```python
from build123d import *

# Parameters (mm, degrees)
EXTRUDE_1_DEPTH   = 7
SKETCH_1_W        = 4.5
SKETCH_1_H        = 2
EXTRUDE_1_2_DEPTH = 7
EXTRUDE_1_3_DEPTH = 7
EXTRUDE_1_4_DEPTH = 7
EXTRUDE_1_5_DEPTH = 7
EXTRUDE_1_6_DEPTH = 7
EXTRUDE_1_7_DEPTH = 7
EXTRUDE_2_DEPTH   = 3
SKETCH_3_W        = 21.86
SKETCH_3_H        = 15
EXTRUDE_3_DEPTH   = 5
FILLET_1_R        = 2
CHAMFER_1_SIZE    = 0.5


with BuildPart() as part:
    # Sketch 1 → Extrude 1 (new body)
    with BuildSketch(Plane(origin=(0, 0, 0), x_dir=(1, 0, 0), z_dir=(0, 1, 0))):
        Polygon((-0.13, 3.475), (-0.13, 1.525), (-2.19, 1.525), (-2.19, -1.525), (-0.13, -1.525), (-0.13, -3.475), (-2.19, -3.475), (-2.19, -6.525), (-0.13, -6.525), (-0.13, -7.495), (1.67, -7.495), (1.67, 7.505), (-0.13, 7.505), (-0.13, 6.525), (-2.19, 6.525), (-2.19, 3.475), align=None)
    extrude(amount=EXTRUDE_1_DEPTH)

    # Sketch 2 → Extrude 2 (add)
    with BuildSketch(Plane(origin=(0, 7, 0), x_dir=(1, 0, 0), z_dir=(0, 1, 0))):
        Polygon((-0.13, 7.505), (-0.13, 6.525), (-2.19, 6.525), (-2.19, 3.475), (-0.13, 3.475), (-0.13, 1.525), (-2.19, 1.525), (-2.19, -1.525), (-0.13, -1.525), (-0.13, -3.475), (-2.19, -3.475), (-2.19, -6.525), (-0.13, -6.525), (-0.13, -7.495), (1.67, -7.495), (1.67, 7.505), align=None)
    extrude(amount=EXTRUDE_2_DEPTH)



with BuildPart() as body_2:
    # Sketch 1 → Extrude 1 2 (new body)
    with BuildSketch(Plane(origin=(0, 0, 0), x_dir=(1, 0, 0), z_dir=(0, 1, 0))):
        with Locations((-7.44, 4)):
            Rectangle(SKETCH_1_W, SKETCH_1_H)
    extrude(amount=EXTRUDE_1_2_DEPTH)


with BuildPart() as body_3:
    # Sketch 1 → Extrude 1 3 (new body)
    with BuildSketch(Plane(origin=(0, 0, 0), x_dir=(1, 0, 0), z_dir=(0, 1, 0))):
        with Locations((-7.44, 0)):
            Rectangle(SKETCH_1_W, SKETCH_1_H)
    extrude(amount=EXTRUDE_1_3_DEPTH)


with BuildPart() as body_4:
    # Sketch 1 → Extrude 1 4 (new body)
    with BuildSketch(Plane(origin=(0, 0, 0), x_dir=(1, 0, 0), z_dir=(0, 1, 0))):
        with Locations((-7.44, -4)):
            Rectangle(SKETCH_1_W, SKETCH_1_H)
    extrude(amount=EXTRUDE_1_4_DEPTH)


with BuildPart() as body_5:
    # Sketch 1 → Extrude 1 5 (new body)
    with BuildSketch(Plane(origin=(0, 0, 0), x_dir=(1, 0, 0), z_dir=(0, 1, 0))):
        with Locations((6.92, 4)):
            Rectangle(SKETCH_1_W, SKETCH_1_H)
    extrude(amount=EXTRUDE_1_5_DEPTH)


with BuildPart() as body_6:
    # Sketch 1 → Extrude 1 6 (new body)
    with BuildSketch(Plane(origin=(0, 0, 0), x_dir=(1, 0, 0), z_dir=(0, 1, 0))):
        with Locations((6.92, 0)):
            Rectangle(SKETCH_1_W, SKETCH_1_H)
    extrude(amount=EXTRUDE_1_6_DEPTH)


with BuildPart() as body_7:
    # Sketch 1 → Extrude 1 7 (new body)
    with BuildSketch(Plane(origin=(0, 0, 0), x_dir=(1, 0, 0), z_dir=(0, 1, 0))):
        with Locations((6.92, -4)):
            Rectangle(SKETCH_1_W, SKETCH_1_H)
    extrude(amount=EXTRUDE_1_7_DEPTH)


with BuildPart() as part_1:
    add(part.part)

    add(body_2.part)  # Extrude 3 merges body 2

    add(body_3.part)  # Extrude 3 merges body 3

    add(body_4.part)  # Extrude 3 merges body 4

    add(body_5.part)  # Extrude 3 merges body 5

    add(body_6.part)  # Extrude 3 merges body 6

    add(body_7.part)  # Extrude 3 merges body 7
    # Sketch 3 → Extrude 3 (add)
    with BuildSketch(Plane.XZ):
        with Locations((-0.26, -0.005)):
            Rectangle(SKETCH_3_W, SKETCH_3_H)
    extrude(amount=EXTRUDE_3_DEPTH)

    # Fillet 1
    fillet_1_edges = [part_1.edges().sort_by_distance(p)[0] for p in [
        (-11.19, -5, -0.005),
        (-0.26, -5, -7.505),
        (10.67, -5, -0.005),
        (-0.26, -5, 7.495),
    ]]
    fillet(fillet_1_edges, radius=FILLET_1_R)

    # Chamfer 1
    chamfer_1_edges = [part_1.edges().sort_by_distance(p)[0] for p in [
        (-5.19, 7, -4),
        (-7.44, 7, -5),
        (-9.69, 7, 0),
        (-7.44, 7, 1),
        (-5.19, 7, 0),
        (-7.44, 7, -1),
        (-9.69, 7, 4),
        (-7.44, 7, 5),
        (-5.19, 7, 4),
        (-7.44, 7, 3),
        (-9.69, 7, -4),
        (4.67, 7, -4),
        (6.92, 7, -3),
        (9.17, 7, -4),
        (6.92, 7, -5),
        (4.67, 7, 0),
        (6.92, 7, 1),
        (9.17, 7, 0),
        (6.92, 7, -1),
        (9.17, 7, 4),
        (6.92, 7, 3),
        (4.67, 7, 4),
        (6.92, 7, 5),
        (-7.44, 7, -3),
        (0.77, 10, -7.505),
        (-0.13, 10, -7.015),
        (-1.16, 10, -6.525),
        (-2.19, 10, -5),
        (-1.16, 10, -3.475),
        (-0.13, 10, -2.5),
        (-1.16, 10, -1.525),
        (-2.19, 10, 0),
        (-1.16, 10, 1.525),
        (-0.13, 10, 2.5),
        (-1.16, 10, 3.475),
        (-2.19, 10, 5),
        (-1.16, 10, 6.525),
        (-0.13, 10, 7.01),
        (0.77, 10, 7.495),
        (1.67, 10, -0.005),
    ]]
    chamfer(chamfer_1_edges, length=CHAMFER_1_SIZE)


solid = part_1.part
```
Work out the finished part from the listing and answer in its coordinate system (mm). A direction names the side the tool comes from. Coordinates: 2 decimals unless noted, no trailing zeros. Order: outer loops, then holes, each group sorted by start corner. A loop starts at its lowest first (then second) coordinate and runs counter-clockwise, first axis right, second up. Notation, with made-up numbers: M 27,53 L 80,53 A11 cw 80,67 Z; hole C -27.5,86.25 d8. An arc over 180 degrees is marked long. Use CSV: the item, a comma, the result in double quotes.
1) Section A-A on z = 0.25 is taken. Write down the section's boundary in (x, y), plus the area to 3 significant figures.
Worked out:
outline,"M -11.19,-3 A2 ccw -9.19,-5 L 8.67,-5 A2 ccw 10.67,-3 L 10.67,0 L 9.17,0 L 9.17,6.5 L 8.67,7 L 5.17,7 L 4.67,6.5 L 4.67,0 L 1.67,0 L 1.67,9.5 L 1.17,10 L -1.69,10 L -2.19,9.5 L -2.19,0 L -5.19,0 L -5.19,6.5 L -5.69,7 L -9.19,7 L -9.69,6.5 L -9.69,0 L -11.19,0 Z"
area,"208 mm^2"
2) Determine the mould class of faces 1 (the face through (-5.19, 3, 0)), 2 (the face through (-1, 5, 6.525)), 3 (the face through (-0.13, 5, 7)), 4 (the face through (10.67, -1, 0)) for opening direction X: released by +X, released by -X, zero draft, split by the parting line, or undercut.
Worked out:
face 1,"undercut"
face 2,"zero draft"
face 3,"released by -X"
face 4,"released by +X"
3) Section C-C on x = -7.5 is taken. Write down the section's boundary in (y, z) (3 decimals).
Worked out:
outline,"M -5,-5.505 A2 ccw -3,-7.505 L 0,-7.505 L 0,-5 L 6.5,-5 L 7,-4.5 L 7,-3.5 L 6.5,-3 L 0,-3 L 0,-1 L 6.5,-1 L 7,-0.5 L 7,0.5 L 6.5,1 L 0,1 L 0,3 L 6.5,3 L 7,3.5 L 7,4.5 L 6.5,5 L 0,5 L 0,7.495 L -3,7.495 A2 ccw -5,5.495 Z"
4) Consider line 1 (Z direction, x = 5, y = 3.5); line 2 (X direction, y = 0.25, z = 0); line 3 (Z direction, x = -1.75, y = 3) (3 decimals). Determine where each line is inside the solid, lowest interval first. Write a range as [from, to].
Worked out:
line 1,"z = [-5, -3], [-1, 1], [3, 5]"
line 2,"x = [-9.69, -5.19], [-2.19, 1.67], [4.67, 9.17]"
line 3,"z = [-6.525, -3.475], [-1.525, 1.525], [3.475, 6.525]"
5) For faces 5 (the face through (7, 3, -1)), 6 (the face through (1.67, 5, 0)), 7 (the face through (-1, 5, -3.475)), 8 (the face through (-7, 3, 3)), 9 (the face through (9.17, 3, -4)), determine the directions among +Z, -Z, +X, -X, +Y, -Y from which every point of the face is accessible in a straight line to the end or side of a thin tool.
Worked out:
face 5,"+X, +Y"
face 6,"+Z, -Z, +Y"
face 7,"+Y"
face 8,"-X, +Y"
face 9,"+Z, -Z, +X, +Y"
6) Flat-ended cylindrical pins translate along their axes: pin 1 Ø1.6 at (y, z) = (2.5, -4) entering from +X; pin 2 Ø1 at (y, z) = (3, 0) entering from -X; pin 3 Ø2.5 at (x, y) = (-6.5, 2) entering from +Z; pin 4 Ø3 at (y, z) = (0.5, -2.5) entering from +X. Find the tip coordinate at first contact, or state that the pin passes through.
Worked out:
pin 1,"stops at x = 9.17"
pin 2,"stops at x = -9.69"
pin 3,"stops at z = 5"
pin 4,"stops at x = 10.67"
7) Section B-B on y = 5 is taken. Count the separate pieces of the cut face and the enclosed holes in it, plus the area to 3 significant figures.
Worked out:
separate pieces,"7"
enclosed holes,"0"
area,"99.8 mm^2"
8) Section D-D on z = -2 is taken. Write down the section's boundary in (x, y), plus the area to 3 significant figures.
Worked out:
outline,"M -11.19,-3 A2 ccw -9.19,-5 L 8.67,-5 A2 ccw 10.67,-3 L 10.67,0 L 1.67,0 L 1.67,9.5 L 1.17,10 L 0.37,10 L -0.13,9.5 L -0.13,0 L -11.19,0 Z"
area,"125 mm^2"
